CAD build for the part. Positions are in the model's coordinates, mm. Face numbers are marked on the shaded views. A direction names the side the tool comes from. Give positions to 0.01 mm unless a question says otherwise; leave off trailing zeros. Loops run counter-clockwise (first coordinate to the right, second up) from the corner with the lowest first, then second, coordinate; pieces in that order, holes last. Notation, with made-up numbers: M 68.25,32.25 L 72.25,32.25 A25 cw 72.25,63.25 Z; hole C 30.25,78 d8. An arc over 180 degrees is marked long. Answer as CSV lines item,"result".
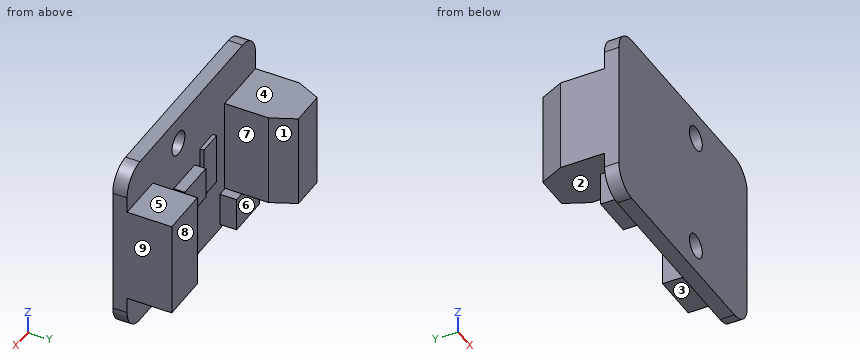
```python
from build123d import *
from OCP.BRepFilletAPI import BRepFilletAPI_MakeChamfer

# Parameters (mm, degrees)
SKETCH1_W           = 30
SKETCH1_H           = 22
BOSS_EXTRUDE1_DEPTH = 1.8
SKETCH2_R           = 1.5
CUT_EXTRUDE1_DEPTH  = 1.8
SKETCH3_W           = 7.2
SKETCH3_H           = 11.8
BOSS_EXTRUDE2_DEPTH = 8.5
SKETCH4_W           = 6
SKETCH4_H           = 12
BOSS_EXTRUDE3_DEPTH = 5.6
SKETCH5_W           = 5.3
SKETCH5_H           = 4.2
BOSS_EXTRUDE4_DEPTH = 2.1
SKETCH6_W           = 4.9
SKETCH6_H           = 4
BOSS_EXTRUDE5_DEPTH = 1.4
SKETCH7_W           = 3
SKETCH7_H           = 6.4
BOSS_EXTRUDE6_DEPTH = 0.5
FILLET1_R           = 3
CHAMFER1_SIZE       = 3
CHAMFER1_SIZE2      = 1.398922974


with BuildPart() as part:
    # Sketch1 → Boss-Extrude1 (new body)
    with BuildSketch(Plane(origin=(0, 0, 0), x_dir=(1, 0, 0), z_dir=(0, 1, 0))):
        with Locations((15, 11)):
            Rectangle(SKETCH1_W, SKETCH1_H)
    extrude(amount=BOSS_EXTRUDE1_DEPTH)

    # Sketch2 → Cut-Extrude1 (cut)
    with BuildSketch(Plane(origin=(0, 1.8, 0), x_dir=(1, 0, 0), z_dir=(0, 1, 0))):
        with Locations(Location((18, 18.5, 0), (0, 0, 270))):
            Circle(SKETCH2_R)
        with Locations(Location((18, 3.5, 0), (0, 0, 270))):
            Circle(SKETCH2_R)
    extrude(amount=-CUT_EXTRUDE1_DEPTH, mode=Mode.SUBTRACT)

    # Sketch3 → Boss-Extrude2 (add)
    with BuildSketch(Plane(origin=(0, 1.8, 0), x_dir=(1, 0, 0), z_dir=(0, 1, 0))):
        with Locations((3.6, 11.2)):
            Rectangle(SKETCH3_W, SKETCH3_H)
    extrude(amount=BOSS_EXTRUDE2_DEPTH)

    # Sketch4 → Boss-Extrude3 (add)
    with BuildSketch(Plane(origin=(0, 1.8, 0), x_dir=(1, 0, 0), z_dir=(0, 1, 0))):
        with Locations((27, 11)):
            Rectangle(SKETCH4_W, SKETCH4_H)
    extrude(amount=BOSS_EXTRUDE3_DEPTH)

    # Sketch5 → Boss-Extrude4 (add)
    with BuildSketch(Plane(origin=(0, 1.8, 0), x_dir=(1, 0, 0), z_dir=(0, 1, 0))):
        with Locations((5.65, 19.3)):
            Rectangle(SKETCH5_W, SKETCH5_H)
    extrude(amount=BOSS_EXTRUDE4_DEPTH)

    # Sketch6 → Boss-Extrude5 (add)
    with BuildSketch(Plane(origin=(0, 1.8, 0), x_dir=(1, 0, 0), z_dir=(0, 1, 0))):
        with Locations((16.65, 11.1)):
            Rectangle(SKETCH6_W, SKETCH6_H)
    extrude(amount=BOSS_EXTRUDE5_DEPTH)

    # Sketch7 → Boss-Extrude6 (add)
    with BuildSketch(Plane(origin=(0, 1.8, 0), x_dir=(1, 0, 0), z_dir=(0, 1, 0))):
        with Locations((11.5, 10.9)):
            Rectangle(SKETCH7_W, SKETCH7_H)
    extrude(amount=BOSS_EXTRUDE6_DEPTH)

    # Fillet1
    fillet1_edges = [part.edges().sort_by_distance(p)[0] for p in [
        (0, 0.9, -22),
        (30, 0.9, -22),
        (30, 0.9, 0),
        (0, 0.9, 0),
    ]]
    fillet(fillet1_edges, radius=FILLET1_R)

    # Chamfer1: one chamfer whose edges measure the first distance from different faces: ONE call of the kernel's chamfer builder (chamfer() names one face for all edges)
    chamfer1_edges_1 = [part.edges().sort_by_distance(p)[0] for p in [
        (0, 10.3, -11.2),
    ]]
    chamfer1_side_1 = [part.faces().sort_by_distance(p)[0] for p in [
        (0, 4.90112316, -11.155383424),
    ]]
    chamfer1_edges_2 = [part.edges().sort_by_distance(p)[0] for p in [
        (7.2, 10.3, -11.2),
    ]]
    chamfer1_side_2 = [part.faces().sort_by_distance(p)[0] for p in [
        (7.2, 6.05, -11.2),
    ]]
    chamfer1 = BRepFilletAPI_MakeChamfer(part.part.solid().wrapped)
    for e in chamfer1_edges_1:
        chamfer1.Add(CHAMFER1_SIZE, CHAMFER1_SIZE2, e.wrapped, chamfer1_side_1[0].wrapped)  # the first distance lies on this face
    for e in chamfer1_edges_2:
        chamfer1.Add(CHAMFER1_SIZE, CHAMFER1_SIZE2, e.wrapped, chamfer1_side_2[0].wrapped)  # the first distance lies on this face
    add(Compound.cast(chamfer1.Shape()), mode=Mode.REPLACE)


solid = part.part
```
Q1. Cut at C-C (z = -14.5). Write the cut outline in (x, y).
Solution:
outline,"M 0,0 L 30,0 L 30,7.4 L 24,7.4 L 24,1.8 L 7.2,1.8 L 7.2,7.3 L 5.8,10.3 L 1.4,10.3 L 0,7.3 Z"
Q2. Cut at A-A (z = -3.5). Write the cut outline in (x, y).
Solution:
outline,"M 0,0 L 16.5,0 L 16.5,1.8 L 0,1.8 Z; M 19.5,0 L 30,0 L 30,1.8 L 19.5,1.8 Z"
Q3. Cut at D-D (x = 24.5). Write the cut outline in (y, z).
Solution:
outline,"M 0,-22 L 1.8,-22 L 1.8,-17 L 7.4,-17 L 7.4,-5 L 1.8,-5 L 1.8,0 L 0,0 Z"
Q4. Mould opens along Z. For the marked faces 1, 2, 3 and 4 say: released by +Z, released by -Z, zero draft, split by the parting line, or undercut.
Solution:
face 1,"zero draft"
face 2,"undercut"
face 3,"released by -Z"
face 4,"released by +Z"
Q5. Wall check: line 1 (X direction, y = 6.75, z = -8.75); line 2 (X direction, y = 0.55, z = -18.5); line 3 (Z direction, x = 18.5, y = 1.75). Give the ranges that are in metal, low to high. Write a range as [from, to].
Solution:
line 1,"x = [0, 7.2], [24, 30]"
line 2,"x = [0, 16.5], [19.5, 30]"
line 3,"z = [-22, -19.91], [-17.09, -4.91], [-2.09, 0]"
Q6. Pin check, flat tips, straight feed: P1, Ø4.5, axis at x = 17.5, z = -10.5, coming from the +Y side; P2, Ø1.8, axis at x = 18, z = -18.5, coming from the +Y side; P3, Ø4.5, axis at x = 26.5, y = 6, coming from the -Z side; P4, Ø3, axis at x = 27.5, y = 3.5, coming from the +Z side. Stop position of each tip, or through.
Solution:
P1,"stops at y = 3.2"
P2,"passes through"
P3,"stops at z = -17"
P4,"stops at z = -5"
Q7. Which spindle directions (+Z, -Z, +X, -X, +Y, -Y) get a long thin tool onto all of the face, cutting with end or side? Do the marked faces 5, 6, 7, 8 and 9. Say none if no direction does.
Solution:
face 5,"+Z, +X, -X, +Y"
face 6,"-Z, +X, -X, +Y"
face 7,"+Z, +Y"
face 8,"+Z, -Z, +X, +Y"
face 9,"+Z, -Z, +X, +Y, -Y"
Q8. Cut at B-B (x = 18). Write the cut outline in (y, z), and give its area (3 significant figures).
Solution:
outline,"M 0,-22 L 1.8,-22 L 1.8,-20 L 0,-20 Z; M 0,-17 L 1.8,-17 L 1.8,-13.1 L 3.2,-13.1 L 3.2,-9.1 L 1.8,-9.1 L 1.8,-5 L 0,-5 Z; M 0,-2 L 1.8,-2 L 1.8,0 L 0,0 Z"
area,"34.4 mm²"
